Autodesk Inventor part; units mm, degrees
ref_plane "YZ Plane" through (0, 0, 0) normal (1, 0, 0) x (0, 1, 0)
ref_plane "XZ Plane" through (0, 0, 0) normal (0, 1, 0) x (-1, 0, 0)
ref_plane "XY Plane" through (0, 0, 0) normal (0, 0, 1) x (1, 0, 0)
sketch "Sketch1" plane through (0, 0, 0) normal (0, 1, 0) x (-1, 0, 0)
  line L0 (-23.3466, 0) -> (-154.4106, 0)
  line L1 (-102.87, 54.61) -> (-74.9238, 54.61)
  line L2 (-88.9, 0) -> (-23.3466, 0)
  line L3 (-88.9, 0) -> (-154.4106, 0)
  arc A0 (-102.87, 54.61) -> (-154.4106, 0) centre (-133.35, 31.75) ccw
  arc A1 (-23.3466, 0) -> (-74.9238, 54.61) centre (-44.4805, 31.7012) ccw
  point P0 (0, 0)
  dimension "d0" = 76.2
  dimension "d1" = 76.2
  dimension "d2" = 131.064
  dimension "d12" = 54.61
extrude "Extrusion1" add sketch "Sketch1" along normal blind 4.826
sketch "Sketch2" plane through (0, 4.826, 0) normal (0, 1, 0) x (1, 0, 0)
  line L0 (154.4106, 0) -> (23.3466, 0)
  arc A0 (23.3466, 0) -> (74.9238, -54.61) centre (44.4805, -31.7012) ccw
  line L1 (74.9238, -54.61) -> (102.87, -54.61)
  arc A1 (102.87, -54.61) -> (154.4106, 0) centre (133.35, -31.75) ccw
  circle A2 centre (44.4805, -31.7012) radius 9.525
  circle A3 centre (133.35, -31.75) radius 9.525
  line L2 (88.8786, 0) -> (88.8969, -54.61)
  line L3 (88.891, -24.1125) -> (88.8786, 0)
  circle A4 centre (132.3699, -12.0338) radius 3
  circle A5 centre (44.4805, -12.0338) radius 3
  circle A6 centre (88.8848, -12.0563) radius 7.5
  point P0 (0, 0)
  dimension "d9" = 6
  dimension "d10" = 6
  dimension "d11" = 15
extrude "Extrusion2" cut sketch "Sketch2" against normal through all contours A6 L2 | L2 A6 | A2 | A3 | A4 | A5
properties part number "paitent remote top"
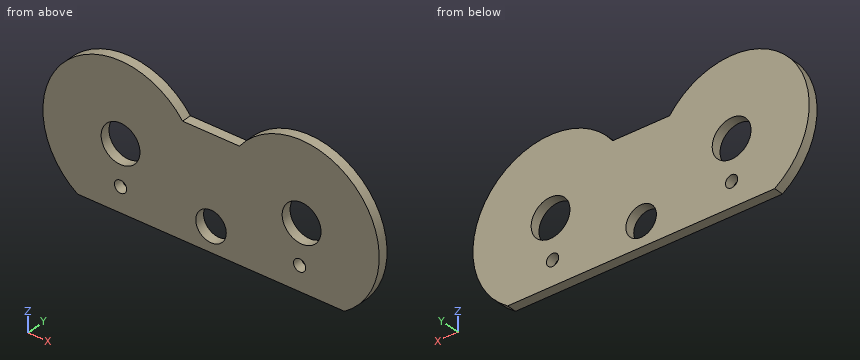
Source: CAD feature listing. Evaluate the final solid. Frame: model axes, mm. Coordinates: 2 decimals unless noted, no trailing zeros. Loops run counter-clockwise (first coordinate to the right, second up) from the corner with the lowest first, then second, coordinate; pieces in that order, holes last. Notation, with made-up numbers: (-25, -32) -> (11, -32) arc R33 cw to (11, 2) -> close; hole circle Ø9 at (-0.5, 38). An arc over 180 degrees is marked (long way). One line per item, written item: value. Start each with the question number.
Q1. Section query C-C, the plane z = 6. Return the cut outline in (x, y), and give its area (3 significant figures).
Q2. Section query D-D, the plane y = 0.95. Give the number of separate pieces and of enclosed holes in the cut face, and give its area (3 significant figures).
Q3. Section query B-B, the plane x = 133.35. Return the cut outline in (y, z) (3 decimals), and give its area (3 significant figures).
Q4. Contact query for flat-ended pins moving along their axis: P1, Ø1.5, axis at y = 2.5, z = 48.5, coming from the -X side; P2, Ø7, axis at x = 44.48, z = 12.03, coming from the -Y side; P3, Ø1.5, axis at y = 3, z = 42.5, coming from the -X side; P4, Ø1, axis at y = 2.5, z = 61, coming from the -X side. Output: stop coordinate, or through.
Q5. Line query: line 1 along X through (y, z) = (4.05, 31); line 2 along X through (y, z) = (0.85, 13); line 3 along X through (y, z) = (3.6, 10.5). Output: solid intervals per line, ascending.
Q6. Section query A-A, the plane z = 35. Return the cut outline in (x, y), and give its area (3 significant figures).
Results:
1. outline: (16.35, 0) -> (84.46, 0) -> (84.46, 4.83) -> (16.35, 4.83) -> close; (93.31, 0) -> (161.43, 0) -> (161.43, 4.83) -> (93.31, 4.83) -> close
1. area: 657 mm^2
2. separate pieces: 1
2. enclosed holes: 5
2. area: 9,080 mm^2
3. outline: (0, 0) -> (4.826, 0) -> (4.826, 9.198) -> (0, 9.198) -> close; (0, 14.869) -> (4.826, 14.869) -> (4.826, 22.225) -> (0, 22.225) -> close; (0, 41.275) -> (4.826, 41.275) -> (4.826, 69.85) -> (0, 69.85) -> close
3. area: 218 mm^2
4. P1: x = 9.93
4. P2: y = 0
4. P3: x = 7.73
4. P4: x = 19.54
5. line 1: 6.39 to 34.98, 53.98 to 123.85, 142.85 to 171.44
5. line 2: 11.29 to 41.64, 47.32 to 81.44, 96.33 to 129.53, 135.21 to 166.52
5. line 3: 12.82 to 41.9, 47.06 to 81.55, 96.22 to 129.79, 134.95 to 164.97
6. outline: (6.52, 0) -> (35.54, 0) -> (35.54, 4.83) -> (6.52, 4.83) -> close; (53.42, 0) -> (124.4, 0) -> (124.4, 4.83) -> (53.42, 4.83) -> close; (142.3, 0) -> (171.31, 0) -> (171.31, 4.83) -> (142.3, 4.83) -> close
6. area: 623 mm^2
